Model file for the job. Use its own axes, mm. A direction names the side the tool comes from. Coordinates: 2 decimals unless noted, no trailing zeros. Loops run counter-clockwise (first coordinate to the right, second up) from the corner with the lowest first, then second, coordinate; pieces in that order, holes last. Notation, with made-up numbers: M 75.5,-18.5 L 100.5,-18.5 A26 cw 100.5,-3.5 Z; hole C 13.5,47 d5. An arc over 180 degrees is marked long. Write item = value, one per line. Start each with the question number.
from build123d import *

# Parameters (mm, degrees)
BASPROSKE_W     = 26
BASPROSKE_H     = 19
TOOTHCUT_DEPTH  = 38.389838192
TEETHCUTS_COUNT = 17
TEETHCUTS_ANGLE = 338.823529412
BORE_DEPTH      = 50.0000508


with BuildPart() as part:
    # BasProSke → Base-Revolve (revolve)
    with BuildSketch(Plane(origin=(0, 0, 0), x_dir=(1, 0, 0), z_dir=(0, 1, 0)), mode=Mode.PRIVATE) as base_revolve_sk:
        with Locations((13, 9.5)):
            Rectangle(BASPROSKE_W, BASPROSKE_H)
    revolve(base_revolve_sk.sketch.rotate(Axis((-10, 0, 0), (1, 0, 0)), 180), axis=Axis((-10, 0, 0), (1, 0, 0)))

    # TooCutSke → ToothCut (cut, through all)
    with BuildSketch(Plane(origin=(0, 0, 0), x_dir=(0, 0, -1), z_dir=(1, 0, 0))):
        with BuildLine():
            ThreePointArc((1.020352389, 14.463052306), (0, 14.499), (-1.020352389, 14.463052306))
            ThreePointArc((-1.020352389, 14.463052306), (-1.632621885, 16.804485203), (-3.026143023, 18.783192049))
            ThreePointArc((-3.026143023, 18.783192049), (0, 19.0254), (3.026143023, 18.783192049))
            ThreePointArc((3.026143023, 18.783192049), (1.632621885, 16.804485203), (1.020352389, 14.463052306))
        make_face()
    toothcut = extrude(amount=TOOTHCUT_DEPTH, mode=Mode.SUBTRACT)

    # TeethCuts: ToothCut ×17 about axis
    teethcuts_axis = Axis((-10, 0, 0), (1, 0, 0))
    for i in range(1, TEETHCUTS_COUNT):
        add(toothcut.rotate(teethcuts_axis, i * TEETHCUTS_ANGLE / (TEETHCUTS_COUNT - 1)), mode=Mode.SUBTRACT)

    # BorSke → Bore (cut, symmetric)
    with BuildSketch(Plane(origin=(0, 0, 0), x_dir=(0, 0, -1), z_dir=(1, 0, 0))):
        with BuildLine():
            Line((-3.55, 2.05121915), (-3.55, -2.05121915))
            ThreePointArc((-3.55, -2.05121915), (2.899137803, -2.899137803), (2.05121915, 3.55))
            Line((2.05121915, 3.55), (-2.05121915, 3.55))
            ThreePointArc((-2.05121915, 3.55), (-2.899137803, 2.899137803), (-3.55, 2.05121915))
        make_face()
    extrude(amount=BORE_DEPTH, both=True, mode=Mode.SUBTRACT)


solid = part.part
Item 1: Probe L1, parallel to Y at x = 20, z = 0; L2, parallel to Z at x = 3, y = 11; L3, parallel to Y at x = 9.25, z = -16.5. List the from-to ranges inside material, lowest first.
Item 2: Cut at A-A (z = 0). Give the cut face in (x, y), plus the area to 3 significant figures.
Item 3: Cut at C-C (y = 10.5). Give the cut face in (x, z) (3 decimals), plus the area to 3 significant figures.
Item 4: Pull direction Y, two halves, no side cores. Call faces 3 (the cylindrical face through (12.818, -3.026, 16.628)), 4 (the cylindrical face through (12.818, 15.092, -7.606)), 5 (the flat face through (26, 4, 0)): +Y half, -Y half, draft (parallel to the pull), parting line (faces both ways), or undercut.
Item 5: Cut at B-B (y = 3). Give the cut face in (x, z).
Item 6: Pin check, flat tips, straight feed: pin 1 Ø8 at (x, y) = (3.5, -11) entering from -Z; pin 2 Ø10 at (x, z) = (6, -11) entering from -Y; pin 3 Ø6.5 at (y, z) = (0, 0) entering from -X; pin 4 Ø6 at (x, y) = (21, 2) entering from -Z. Stop position of each tip, or through.
Item 7: 3-axis set-ups, long thin cutter, end or side, ignore diameter. For faces 1 (the cylindrical face through (12.82, 6.48, 12.97)), 2 (the cylindrical face through (12.818, 11.326, -12.544)): which of +Z, -Z, +X, -X, +Y, -Y reach the whole face in a straight line?
Item 8: Cut at D-D (y = -6.5). Give the cut face in (x, z), plus the area to 3 significant figures.
Reported:
q1.L1 = -19 to -4.1, 3.55 to 14.5
q1.L2 = -15.44 to -11.87, -9.45 to 9.45, 11.87 to 15.44
q1.L3 = -8.94 to -6.97, -3.04 to 0.05, 3.13 to 6.01
q2.outline = M 0,-19 L 26,-19 L 26,-4.1 L 0,-4.1 Z; M 0,3.55 L 26,3.55 L 26,14.5 L 0,14.5 Z
q2.area = 672 mm^2
q3.outline = M 0,-15.245 L 26,-15.245 L 26,-11.093 L 0,-11.093 Z; M 0,-9.999 L 26,-9.999 L 26,9.999 L 0,9.999 Z; M 0,11.093 L 26,11.093 L 26,15.245 L 0,15.245 Z
q3.area = 736 mm^2
q4.face_3 = undercut
q4.face_4 = +Y half
q4.face_5 = draft
q5.outline = M 0,-16.26 L 26,-16.26 L 26,-2.79 L 0,-2.79 Z; M 0,2.79 L 26,2.79 L 26,16.26 L 0,16.26 Z
q6.pin_1 = -17.22
q6.pin_2 = -17.89
q6.pin_3 = through
q6.pin_4 = -18.63
q7.face_1 = +X, -X
q7.face_2 = +X, -X, +Y
q8.outline = M 0,-16.07 L 26,-16.07 L 26,16.07 L 0,16.07 Z
q8.area = 836 mm^2
